Part print with two shaded views. Sizes in mm from the minimum x, y, z corner. Give positions to 0.01 mm unless a question says otherwise; leave off trailing zeros. Order: outer loops, then holes, each group sorted by start corner. A loop starts at its lowest first (then second) coordinate and runs counter-clockwise, first axis right, second up.
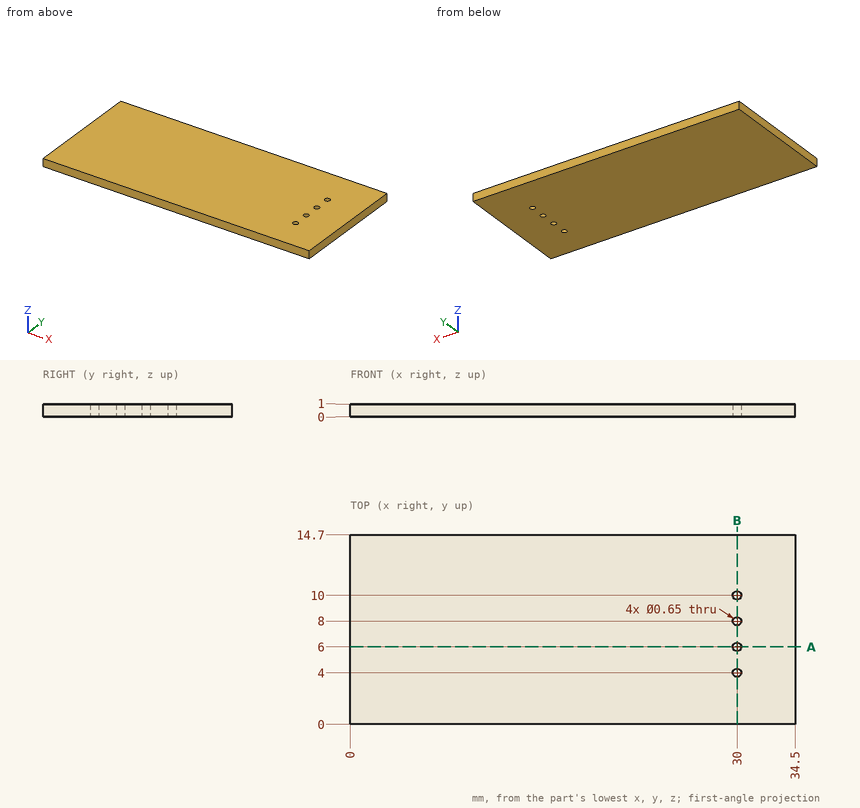
1. Saw through at B-B on x = 30. Give the cut face in (y, z) (3 decimals).
2. Saw through at A-A on y = 6. Give the cut face in (x, z) (3 decimals), plus the area to 4 significant figures.
3. Wall check: line 1 (Y direction, x = 30, z = 0.4) (3 decimals); line 2 (X direction, y = 8, z = 0.25) (3 decimals). Give the ranges that are in metal, low to high.
Reported:
1. outline: (0, 0) - (3.675, 0) - (3.675, 1) - (0, 1) - close; (4.325, 0) - (5.675, 0) - (5.675, 1) - (4.325, 1) - close; (6.325, 0) - (7.675, 0) - (7.675, 1) - (6.325, 1) - close; (8.325, 0) - (9.675, 0) - (9.675, 1) - (8.325, 1) - close; (10.325, 0) - (14.7, 0) - (14.7, 1) - (10.325, 1) - close
2. outline: (0, 0) - (29.675, 0) - (29.675, 1) - (0, 1) - close; (30.325, 0) - (34.5, 0) - (34.5, 1) - (30.325, 1) - close
2. area: 33.85 mm2
3. line 1: y = 0 to 3.675, 4.325 to 5.675, 6.325 to 7.675, 8.325 to 9.675, 10.325 to 14.7
3. line 2: x = 0 to 29.675, 30.325 to 34.5
